from build123d import *

# Parameters (mm, degrees)
F1_DEPTH = 25


with BuildPart() as f1:
    # F0 (on Front) → F1 (new body, symmetric)
    with BuildSketch(Plane.XZ):
        Polygon((-43.168996, 6), (-43.168996, 0), (-23.168996, 0), (-23.168996, 6), (-29.168996, 6), (-29.168996, 31.558661), (-5.5, 0), (0.619155, 0), (9.011236, 11.700977), (9.011236, 3), (6.011236, 3), (6.011236, 0), (16.011236, 0), (16.011236, 3), (13.011236, 3), (13.011236, 15.775682), (7.011236, 15.775682), (0, 6), (-25.168996, 39.558661), (-37.168996, 39.558661), (-37.168996, 6), align=None)
    extrude(amount=F1_DEPTH, both=True)


solid = f1.part
Design review of the part built by this model. Coordinates are the model's own, in mm. A direction names the side the tool comes from. Coordinates: 2 decimals unless noted, no trailing zeros. Loops run counter-clockwise (first coordinate to the right, second up) from the corner with the lowest first, then second, coordinate; pieces in that order, holes last. Notation, with made-up numbers: (3.25, 53.25) -> (44.25, 53.25) arc R32 cw to (44.25, 82.25) -> close; hole circle Ø2 at (-19, 40.5). An arc over 180 degrees is marked (long way). Use a Markdown table: item, result. Add a question column.
Item 1: We need section A-A, the plane z = 22.5. Write out the cut boundary in (x, y) (3 decimals).
Item 2: We need section D-D, the plane x = -12. Write out the cut boundary in (y, z), and give its area (3 significant figures).
Item 3: Machinability: for faces 4 (the flat face through (-40, 0, 6)), 5 (the flat face through (13.011, 0, 9)), 6 (the flat face through (-17.5, -0.4, 16)), which of the approach directions +Z, -Z, +X, -X, +Y, -Y give a long, thin tool a straight path to every point of the face, cutting with its end or side? Answer none if there is none.
Item 4: We need section B-B, the plane y = -16. Write out the cut boundary in (x, z).
Item 5: The part is to be moulded in two halves that separate along X. For faces 1 (the flat face through (16.011, 0, 1)), 2 (the flat face through (15, 0, 3)), 3 (the flat face through (6.011, 0, 2)), say which applies: +X half, -X half, draft (parallel to the pull), parting line (faces both ways), or undercut.
Item 6: Wall thickness on L1, parallel to X at y = 12, z = 4.5 (3 decimals); L2, parallel to X at y = -1, z = 11; L3, parallel to X at y = -10.5, z = 14: over which ranges is each line inside the solid? List them lowest first. Write a range as from..to.
Item 7: Clearance check with flat-ended pins moving along their axes: P1, Ø10, axis at y = 3.5, z = 29, coming from the -X side; P2, Ø6.5, axis at y = 6, z = 8, coming from the +X side; P3, Ø6.5, axis at x = 10.5, y = 9, coming from the +Z side; P4, Ø8, axis at x = -15, z = 32.5, coming from the -Y side. State where each tip first meets the part, or that it passes through.
Item 8: We need section C-C, the plane z = 8. Write out the cut boundary in (x, y), and give its area (3 significant figures).
Numbers:
| question | item | result |
|---|---|---|
| 1 | outline | (-37.169, -25) -> (-29.169, -25) -> (-29.169, 25) -> (-37.169, 25) -> close; (-22.375, -25) -> (-12.375, -25) -> (-12.375, 25) -> (-22.375, 25) -> close |
| 2 | outline | (-25, 8.67) -> (25, 8.67) -> (25, 22) -> (-25, 22) -> close |
| 2 | area | 667 mm^2 |
| 3 | face 4 | +Z, -X, +Y, -Y |
| 3 | face 5 | +Z, +X, +Y, -Y |
| 3 | face 6 | +Y, -Y |
| 4 | outline | (-43.17, 0) -> (-23.17, 0) -> (-23.17, 6) -> (-29.17, 6) -> (-29.17, 31.56) -> (-5.5, 0) -> (0.62, 0) -> (9.01, 11.7) -> (9.01, 3) -> (6.01, 3) -> (6.01, 0) -> (16.01, 0) -> (16.01, 3) -> (13.01, 3) -> (13.01, 15.78) -> (7.01, 15.78) -> (0, 6) -> (-25.17, 39.56) -> (-37.17, 39.56) -> (-37.17, 6) -> (-43.17, 6) -> close |
| 5 | face 1 | +X half |
| 5 | face 2 | draft |
| 5 | face 3 | undercut |
| 6 | L1 | x = -43.169..-23.169, -8.875..3.847, 9.011..13.011 |
| 6 | L2 | x = -37.17..-29.17, -13.75..-3.75, 3.59..8.51, 9.01..13.01 |
| 6 | L3 | x = -37.17..-29.17, -16..-6, 5.74..13.01 |
| 7 | P1 | stops at x = -37.17 |
| 7 | P2 | stops at x = 13.01 |
| 7 | P3 | stops at z = 15.78 |
| 7 | P4 | stops at y = -25 |
| 8 | outline | (-37.17, -25) -> (-29.17, -25) -> (-29.17, 25) -> (-37.17, 25) -> close; (-11.5, -25) -> (-1.5, -25) -> (-1.5, 25) -> (-11.5, 25) -> close; (1.43, -25) -> (6.36, -25) -> (6.36, 25) -> (1.43, 25) -> close; (9.01, -25) -> (13.01, -25) -> (13.01, 25) -> (9.01, 25) -> close |
| 8 | area | 1,350 mm^2 |
